```python
from build123d import *

# Parameters (mm, degrees)
SALIENTE_EXTRUIR1_DEPTH = 100
CROQUIS3_R              = 7.5
CROQUIS3_R_2            = 15
CROQUIS3_R_3            = 22.5
CORTAR_EXTRUIR1_DEPTH   = 226.610283454
CHAFL_N1_SIZE           = 5


with BuildPart() as part:
    # Croquis2 → Saliente-Extruir1 (new body)
    with BuildSketch(Plane.XY):
        Polygon((10, 30), (190, 30), (200, 20), (200, 10), (190, 0), (10, 0), (0, 10), (0, 20), align=None)
    extrude(amount=-SALIENTE_EXTRUIR1_DEPTH)

    # Croquis3 → Cortar-Extruir1 (cut, through all)
    with BuildSketch(Plane(origin=(0, 30, 0), x_dir=(1, 0, 0), z_dir=(0, 1, 0))):
        with Locations(Location((25, 50, 0), (0, 0, 270))):
            Circle(CROQUIS3_R)
        with Locations(Location((75, 50, 0), (0, 0, 270))):
            Circle(CROQUIS3_R_2)
        with Locations(Location((150, 50, 0), (0, 0, 270))):
            Circle(CROQUIS3_R_3)
    extrude(amount=-CORTAR_EXTRUIR1_DEPTH, mode=Mode.SUBTRACT)

    # Chaflán1
    chafl_n1_edges = [part.edges().sort_by_distance(p)[0] for p in [
        (25, 30, -57.5),
        (75, 30, -65),
        (150, 30, -72.5),
    ]]
    chamfer(chafl_n1_edges, length=CHAFL_N1_SIZE)


solid = part.part
```
Geometry: final body of the model. Coordinates: model frame, mm. Round coordinates to 2 decimals unless told otherwise and drop trailing zeros. Order: outer loops, then holes, each group sorted by start corner. A loop starts at its lowest first (then second) coordinate and runs counter-clockwise, first axis right, second up. Notation, with made-up numbers: (35, 16.5) - (81, 16.5) arc R20 cw to (81, 47.5) - close; hole circle Ø3 at (-11, 18). An arc over 180 degrees is marked (long way). Write item = value, one per line. Start each with the question number.
Q1. Ray query, line 1 (X direction, y = 6, z = -39.5); line 2 (X direction, y = 11.5, z = -40.5); line 3 (X direction, y = 7, z = -50). Return the intervals inside material, ascending. Write a range as from..to.
Q2. Cut plane D-D on x = 25. Return the cut outline in (y, z), and give its area (4 significant figures).
Q3. Cut plane B-B on z = -50. Return the cut outline in (x, y).
Q4. Pull-direction query (Z, two-part tool) for faces 1 (the flat face through (5, 25, -49)), 2 (the cylindrical face through (60.357, 12.675, -53.252)), 3 (the flat face through (101, 15, 0)), 4 (the cylindrical face through (31.324, 12.675, -45.968)); classes: +Z half, -Z half, draft (parallel to the pull), parting line (faces both ways), or undercut.
Q5. Cut plane C-C on y = 8. Return the cut outline in (x, z).
Q6. Cut plane A-A on x = 150. Return the cut outline in (y, z), and give its area (4 significant figures).
Outcome:
q1.line_1 = 4..64.29, 85.71..130.1, 169.9..196
q1.line_2 = 0..63.39, 86.61..129.6, 170.4..200
q1.line_3 = 3..17.5, 32.5..60, 90..127.5, 172.5..197
q2.outline = (0, -100) - (30, -100) - (30, -62.5) - (25, -57.5) - (0, -57.5) - close; (0, -42.5) - (25, -42.5) - (30, -37.5) - (30, 0) - (0, 0) - close
q2.area = 2,525 mm^2
q3.outline = (0, 10) - (10, 0) - (17.5, 0) - (17.5, 25) - (12.5, 30) - (10, 30) - (0, 20) - close; (32.5, 0) - (60, 0) - (60, 25) - (55, 30) - (37.5, 30) - (32.5, 25) - close; (90, 0) - (127.5, 0) - (127.5, 25) - (122.5, 30) - (95, 30) - (90, 25) - close; (172.5, 0) - (190, 0) - (200, 10) - (200, 20) - (190, 30) - (177.5, 30) - (172.5, 25) - close
q4.face_1 = draft
q4.face_2 = undercut
q4.face_3 = +Z half
q4.face_4 = undercut
q5.outline = (2, -100) - (198, -100) - (198, 0) - (2, 0) - close; hole circle Ø15 at (25, -50); hole circle Ø30 at (75, -50); hole circle Ø45 at (150, -50)
q6.outline = (0, -100) - (30, -100) - (30, -77.5) - (25, -72.5) - (0, -72.5) - close; (0, -27.5) - (25, -27.5) - (30, -22.5) - (30, 0) - (0, 0) - close
q6.area = 1,625 mm^2
